Source: CAD feature listing. Evaluate the final solid. Frame: model axes, mm. A direction names the side the tool comes from. Give positions to 0.01 mm unless a question says otherwise; leave off trailing zeros. Order: outer loops, then holes, each group sorted by start corner. A loop starts at its lowest first (then second) coordinate and runs counter-clockwise, first axis right, second up. Notation, with made-up numbers: M 86,51 L 130,51 A22 ccw 130,89 Z; hole C 77,86.25 d9. An arc over 180 degrees is marked long. Use CSV: the item, a comma, the result in double quotes. Start each with the question number.
1. Pin query (flat end, axial travel): P1, Ø1, axis at x = 22.5, y = 1.5, coming from the +Z side; P2, Ø0.6, axis at y = 1, z = -22, coming from the +X side; P3, Ø1, axis at y = 0.5, z = -30.5, coming from the +X side. Return the tip coordinate at first contact, or that it passes through.
2. Section query B-B, the plane z = 16. Return the cut outline in (x, y), plus the area to 3 significant figures.
3. Section query C-C, the plane x = 12. Return the cut outline in (y, z), plus the area to 3 significant figures.
4. Section query A-A, the plane x = -15. Return the cut outline in (y, z), plus the area to 3 significant figures.
5. Section query D-D, the plane y = 0.65. State how many separate pieces and enclosed holes the cut face has, plus the area to 3 significant figures.
6. Line query: line 1 along X through (y, z) = (0.6, -5); line 2 along Z through (x, y) = (35, 0.3); line 3 along Z through (x, y) = (-17.5, 0.25). Output: solid intervals per line, ascending. Write a range as [from, to].
7. Reachability of faces 1 (the flat face through (-16, 1, -10.33)), 2 (the flat face through (8.642, 1, -27)), 3 (the flat face through (34, 1, 13.92)), 4 (the flat face through (-33, 1, 13.92)) from +Z, -Z, +X, -X, +Y, -Y: full face, straight path, thin tool, end or side. Return the list, or none.
from build123d import *

# Parameters (mm, degrees)
SKETCH1_R           = 1.5
BOSS_EXTRUDE1_DEPTH = 2
CUT_EXTRUDE1_DEPTH  = 2
FILLET1_R           = 2
SKETCH3_R           = 2.5
CUT_EXTRUDE2_DEPTH  = 10


with BuildPart() as part:
    # Sketch1 → Boss-Extrude1 (new body)
    with BuildSketch(Plane(origin=(0, 0, 0), x_dir=(1, 0, 0), z_dir=(0, 1, 0))):
        with BuildLine():
            Line((8.64173402, -21.920230415), (8.64173402, -9.920230415))
            Line((8.64173402, -9.920230415), (30.694037343, -9.920230415))
            Line((30.694037343, -9.920230415), (30.694037343, -13.920230415))
            Line((30.694037343, -13.920230415), (36.694037343, -13.920230415))
            Line((36.694037343, -13.920230415), (36.694037343, -9.920230415))
            ThreePointArc((36.694037343, -9.920230415), (43.39173402, 5.329769585), (36.694037343, 20.579769585))
            Line((36.694037343, 20.579769585), (36.694037343, 24.579769585))
            Line((36.694037343, 24.579769585), (30.694037343, 24.579769585))
            Line((30.694037343, 24.579769585), (30.694037343, 20.579769585))
            Line((30.694037343, 20.579769585), (8.64173402, 20.579769585))
            Line((8.64173402, 20.579769585), (8.64173402, 34.579769585))
            Line((8.64173402, 34.579769585), (-8.35826598, 34.579769585))
            Line((-8.35826598, 34.579769585), (-8.35826598, 20.579769585))
            Line((-8.35826598, 20.579769585), (-30.410569302, 20.579769585))
            Line((-30.410569302, 20.579769585), (-30.410569302, 24.579769585))
            Line((-30.410569302, 24.579769585), (-36.410569302, 24.579769585))
            Line((-36.410569302, 24.579769585), (-36.410569302, 20.579769585))
            ThreePointArc((-36.410569302, 20.579769585), (-43.10826598, 5.329769585), (-36.410569302, -9.920230415))
            Line((-36.410569302, -9.920230415), (-36.410569302, -13.920230415))
            Line((-36.410569302, -13.920230415), (-30.410569302, -13.920230415))
            Line((-30.410569302, -13.920230415), (-30.410569302, -9.920230415))
            Line((-30.410569302, -9.920230415), (-8.35826598, -9.920230415))
            Line((-8.35826598, -9.920230415), (-8.35826598, -21.920230415))
            Line((-8.35826598, -21.920230415), (8.64173402, -21.920230415))
        make_face()
        with Locations(Location((-33.410569302, 21.579769585, 0), (0, 0, 270))):
            Circle(SKETCH1_R, mode=Mode.SUBTRACT)
        with Locations(Location((-33.410569302, -10.920230415, 0), (0, 0, 270))):
            Circle(SKETCH1_R, mode=Mode.SUBTRACT)
        with Locations(Location((33.694037343, -10.920230415, 0), (0, 0, 270))):
            Circle(SKETCH1_R, mode=Mode.SUBTRACT)
        with Locations(Location((33.694037343, 21.579769585, 0), (0, 0, 270))):
            Circle(SKETCH1_R, mode=Mode.SUBTRACT)
    extrude(amount=BOSS_EXTRUDE1_DEPTH)

    # Sketch2 → Cut-Extrude1 (cut)
    with BuildSketch(Plane(origin=(0, 2, 0), x_dir=(1, 0, 0), z_dir=(0, 1, 0))):
        with BuildLine():
            Line((-24.10826598, 10.329769585), (-8.10826598, 10.329769585))
            ThreePointArc((-8.10826598, 10.329769585), (-3.10826598, 5.329769585), (-8.10826598, 0.329769585))
            Line((-8.10826598, 0.329769585), (-24.10826598, 0.329769585))
            ThreePointArc((-24.10826598, 0.329769585), (-29.10826598, 5.329769585), (-24.10826598, 10.329769585))
        make_face()
    extrude(amount=-CUT_EXTRUDE1_DEPTH, mode=Mode.SUBTRACT)

    # Fillet1
    fillet1_edges = [part.edges().sort_by_distance(p)[0] for p in [
        (-30.410569302, 1, 13.920230415),
        (-36.410569302, 1, 13.920230415),
        (-36.410569302, 1, -24.579769585),
        (-30.410569302, 1, -24.579769585),
        (30.694037343, 1, -24.579769585),
        (36.694037343, 1, -24.579769585),
        (36.694037343, 1, 13.920230415),
        (30.694037343, 1, 13.920230415),
    ]]
    fillet(fillet1_edges, radius=FILLET1_R)

    # Sketch3 → Cut-Extrude2 (cut)
    with BuildSketch(Plane.XZ):
        with Locations(Location((0.14173402, -27.579769585, 0), (0, 0, 270))):
            Circle(SKETCH3_R)
        with Locations(Location((0.14173402, 15.920230415, 0), (0, 0, 270))):
            Circle(SKETCH3_R)
    extrude(amount=-CUT_EXTRUDE2_DEPTH, mode=Mode.SUBTRACT)


solid = part.part
Result set:
1,P1,"z = 9.92"
1,P2,"x = 36.69"
1,P3,"x = 8.64"
2,outline,"M -8.36,0 L -2.36,0 L -2.36,2 L -8.36,2 Z; M 2.64,0 L 8.64,0 L 8.64,2 L 2.64,2 Z"
2,area,"24.0 mm2"
3,outline,"M 0,-20.58 L 2,-20.58 L 2,9.92 L 0,9.92 Z"
3,area,"61.0 mm2"
4,outline,"M 0,-20.58 L 2,-20.58 L 2,-10.33 L 0,-10.33 Z; M 0,-0.33 L 2,-0.33 L 2,9.92 L 0,9.92 Z"
4,area,"41.0 mm2"
5,separate pieces,"1"
5,enclosed holes,"7"
5,area,"2,740 mm2"
6,line 1,"[-43.11, -29.1], [-3.12, 43.39]"
6,line 2,"[-24.56, -22.32], [-20.84, 10.18], [11.66, 13.9]"
6,line 3,"[-20.58, -10.33], [-0.33, 9.92]"
7,face 1,"+Y, -Y"
7,face 2,"-Z, +Y, -Y"
7,face 3,"+Z, +X, +Y, -Y"
7,face 4,"+Z, -X, +Y, -Y"
